Work out the finished part from the listing and answer in its coordinate system (mm). A direction names the side the tool comes from. Give positions to 0.01 mm unless a question says otherwise; leave off trailing zeros. Write each loop counter-clockwise with the first axis right and the second up, starting at its lowest first coordinate (ties: lowest second). Pieces come first, ordered by that corner, then holes. Notation, with made-up numbers: (57.5, -37) -> (95.5, -37) arc R16 ccw to (95.5, -17) -> close; hole circle Ø6 at (38.25, 33.5). An arc over 180 degrees is marked (long way). Use a Markdown table: item, result. Add a question column.
Q1. Consider line 1 (Y direction, x = -40, z = 2.9); line 2 (Y direction, x = 0, z = 3.45); line 3 (X direction, y = 20, z = 3.1). Determine where each line is inside the solid, lowest interval first.
Q2. Section D-D, the plane y = -21.5 is taken. Give the vertices of the cut face in (x, z).
Q3. Section A-A, the plane x = -40 is taken. Give the vertices of the cut face in (y, z), plus the area to 3 significant figures.
Q4. Each of these flat-tipped pins is pushed along its axis until it touches: pin 1 Ø6 at (x, y) = (28.5, -12.5) entering from -Z; pin 2 Ø2.5 at (x, z) = (-38.5, 3) entering from +Y; pin 3 Ø3.5 at (x, y) = (30.5, 30.5) entering from -Z (3 decimals); pin 4 Ø1.5 at (x, z) = (40.5, 2) entering from -Y. Where does it stop, or does it pass through?
Q5. Section B-B, the plane x = 0 is taken. Give the vertices of the cut face in (y, z), plus the area to 3 significant figures.
Q6. For a pull along X with two mould halves and no side action, classify faces 4 (the face through (0, -45, 2)), 5 (the face through (33, -40, 2)), 6 (the face through (-29.577, 28.726, 2.465)) as pulls with the +X half, pulls with the -X half, needs draft (parallel to the pull), parting line crosses it, or undercut.
Q7. Section C-C, the plane z = 1.8 is taken. State how many separate pieces and enclosed holes the cut face has, plus the area to 3 significant figures.
Q8. For faces 1 (the face through (40, 33, 2)), 2 (the face through (-41, 33, 2)), 3 (the face through (-40, -33, 2)), determine the directions among +Z, -Z, +X, -X, +Y, -Y from which every point of the face is accessible in a straight line to the end or side of a thin tool.
from build123d import *

# Parameters (mm, degrees)
SKETCH1_R           = 30.5
SKETCH1_R_2         = 2
BOSS_EXTRUDE1_DEPTH = 5
FILLET1_R           = 3
CUT_EXTRUDE1_REACH  = 65.836
SKETCH2_R           = 2


with BuildPart() as part:
    # Sketch1 → Boss-Extrude1 (new body)
    with BuildSketch(Plane.XY):
        Polygon((33, -45), (-33, -45), (-33, -33), (-45, -33), (-45, 33), (-33, 33), (-33, 45), (33, 45), (33, 33), (45, 33), (45, -33), (33, -33), align=None)
        Circle(SKETCH1_R, mode=Mode.SUBTRACT)
        with Locations((-30.5, 30.5)):
            Circle(SKETCH1_R_2, mode=Mode.SUBTRACT)
        with Locations(Location((30.5, 30.5, 0), (0, 0, 180))):
            Circle(SKETCH1_R_2, mode=Mode.SUBTRACT)
        with Locations((30.5, -30.5)):
            Circle(SKETCH1_R_2, mode=Mode.SUBTRACT)
        with Locations(Location((-30.5, -30.5, 0), (0, 0, 180))):
            Circle(SKETCH1_R_2, mode=Mode.SUBTRACT)
    extrude(amount=BOSS_EXTRUDE1_DEPTH)

    # Fillet1
    fillet1_edges = [part.edges().sort_by_distance(p)[0] for p in [
        (33, 33, 2.5),
        (33, -33, 2.5),
        (-33, -33, 2.5),
        (-33, 33, 2.5),
    ]]
    fillet(fillet1_edges, radius=FILLET1_R)

    # Sketch2 → Cut-Extrude1 (cut, up to next)
    with BuildSketch(Plane(origin=(0, 0, 0), x_dir=(-1, 0, 0), z_dir=(0, 0, -1)), mode=Mode.PRIVATE) as cut_extrude1_sk1:
        with Locations((-25, 40)):
            Circle(SKETCH2_R)
    cut_extrude1_tool1 = extrude(cut_extrude1_sk1.sketch, amount=-CUT_EXTRUDE1_REACH, mode=Mode.PRIVATE) & part.part
    # Sketch2 → Cut-Extrude1 (cut, up to next)
    with BuildSketch(Plane(origin=(0, 0, 0), x_dir=(-1, 0, 0), z_dir=(0, 0, -1)), mode=Mode.PRIVATE) as cut_extrude1_sk2:
        with Locations((40, 25)):
            Circle(SKETCH2_R)
    cut_extrude1_tool2 = extrude(cut_extrude1_sk2.sketch, amount=-CUT_EXTRUDE1_REACH, mode=Mode.PRIVATE) & part.part
    # Sketch2 → Cut-Extrude1 (cut, up to next)
    with BuildSketch(Plane(origin=(0, 0, 0), x_dir=(-1, 0, 0), z_dir=(0, 0, -1)), mode=Mode.PRIVATE) as cut_extrude1_sk3:
        with Locations((25, 40)):
            Circle(SKETCH2_R)
    cut_extrude1_tool3 = extrude(cut_extrude1_sk3.sketch, amount=-CUT_EXTRUDE1_REACH, mode=Mode.PRIVATE) & part.part
    # Sketch2 → Cut-Extrude1 (cut, up to next)
    with BuildSketch(Plane(origin=(0, 0, 0), x_dir=(-1, 0, 0), z_dir=(0, 0, -1)), mode=Mode.PRIVATE) as cut_extrude1_sk4:
        with Locations((25, -40)):
            Circle(SKETCH2_R)
    cut_extrude1_tool4 = extrude(cut_extrude1_sk4.sketch, amount=-CUT_EXTRUDE1_REACH, mode=Mode.PRIVATE) & part.part
    # Sketch2 → Cut-Extrude1 (cut, up to next)
    with BuildSketch(Plane(origin=(0, 0, 0), x_dir=(-1, 0, 0), z_dir=(0, 0, -1)), mode=Mode.PRIVATE) as cut_extrude1_sk5:
        with Locations((-25, -40)):
            Circle(SKETCH2_R)
    cut_extrude1_tool5 = extrude(cut_extrude1_sk5.sketch, amount=-CUT_EXTRUDE1_REACH, mode=Mode.PRIVATE) & part.part
    # Sketch2 → Cut-Extrude1 (cut, up to next)
    with BuildSketch(Plane(origin=(0, 0, 0), x_dir=(-1, 0, 0), z_dir=(0, 0, -1)), mode=Mode.PRIVATE) as cut_extrude1_sk6:
        with Locations((40, -25)):
            Circle(SKETCH2_R)
    cut_extrude1_tool6 = extrude(cut_extrude1_sk6.sketch, amount=-CUT_EXTRUDE1_REACH, mode=Mode.PRIVATE) & part.part
    # Sketch2 → Cut-Extrude1 (cut, up to next)
    with BuildSketch(Plane(origin=(0, 0, 0), x_dir=(-1, 0, 0), z_dir=(0, 0, -1)), mode=Mode.PRIVATE) as cut_extrude1_sk7:
        with Locations((-40, 25)):
            Circle(SKETCH2_R)
    cut_extrude1_tool7 = extrude(cut_extrude1_sk7.sketch, amount=-CUT_EXTRUDE1_REACH, mode=Mode.PRIVATE) & part.part
    # Sketch2 → Cut-Extrude1 (cut, up to next)
    with BuildSketch(Plane(origin=(0, 0, 0), x_dir=(-1, 0, 0), z_dir=(0, 0, -1)), mode=Mode.PRIVATE) as cut_extrude1_sk8:
        with Locations((-40, -25)):
            Circle(SKETCH2_R)
    cut_extrude1_tool8 = extrude(cut_extrude1_sk8.sketch, amount=-CUT_EXTRUDE1_REACH, mode=Mode.PRIVATE) & part.part
    add(cut_extrude1_tool1.solids().sort_by_distance((25, 40, 0))[0], mode=Mode.SUBTRACT)
    add(cut_extrude1_tool2.solids().sort_by_distance((-40, 25, 0))[0], mode=Mode.SUBTRACT)
    add(cut_extrude1_tool3.solids().sort_by_distance((-25, 40, 0))[0], mode=Mode.SUBTRACT)
    add(cut_extrude1_tool4.solids().sort_by_distance((-25, -40, 0))[0], mode=Mode.SUBTRACT)
    add(cut_extrude1_tool5.solids().sort_by_distance((25, -40, 0))[0], mode=Mode.SUBTRACT)
    add(cut_extrude1_tool6.solids().sort_by_distance((-40, -25, 0))[0], mode=Mode.SUBTRACT)
    add(cut_extrude1_tool7.solids().sort_by_distance((40, 25, 0))[0], mode=Mode.SUBTRACT)
    add(cut_extrude1_tool8.solids().sort_by_distance((40, -25, 0))[0], mode=Mode.SUBTRACT)


solid = part.part
Result set:
| question | item | result |
|---|---|---|
| 1 | line 1 | y = -33 to -27, -23 to 23, 27 to 33 |
| 1 | line 2 | y = -45 to -30.5, 30.5 to 45 |
| 1 | line 3 | x = -45 to -23.03, 23.03 to 45 |
| 2 | outline | (-45, 0) -> (-21.63, 0) -> (-21.63, 5) -> (-45, 5) -> close; (21.63, 0) -> (45, 0) -> (45, 5) -> (21.63, 5) -> close |
| 3 | outline | (-33, 0) -> (-27, 0) -> (-27, 5) -> (-33, 5) -> close; (-23, 0) -> (23, 0) -> (23, 5) -> (-23, 5) -> close; (27, 0) -> (33, 0) -> (33, 5) -> (27, 5) -> close |
| 3 | area | 290 mm2 |
| 4 | pin 1 | stops at z = 0 |
| 4 | pin 2 | stops at y = 33 |
| 4 | pin 3 | passes through |
| 4 | pin 4 | stops at y = -33 |
| 5 | outline | (-45, 0) -> (-30.5, 0) -> (-30.5, 5) -> (-45, 5) -> close; (30.5, 0) -> (45, 0) -> (45, 5) -> (30.5, 5) -> close |
| 5 | area | 145 mm2 |
| 6 | face 4 | needs draft |
| 6 | face 5 | pulls with the +X half |
| 6 | face 6 | undercut |
| 7 | separate pieces | 1 |
| 7 | enclosed holes | 13 |
| 7 | area | 4,460 mm2 |
| 8 | face 1 | +Z, -Z, +X, +Y |
| 8 | face 2 | +Z, -Z, -X, +Y |
| 8 | face 3 | +Z, -Z, -X, -Y |
